Work out the finished part from the listing and answer in its coordinate system (mm). Face numbers are marked on the shaded views. Coordinates: 2 decimals unless noted, no trailing zeros. Loops run counter-clockwise (first coordinate to the right, second up) from the corner with the lowest first, then second, coordinate; pieces in that order, holes last. Notation, with made-up numbers: (-7, 12) - (2, 12) arc R17 ccw to (2, 31) - close; hole circle Ø5 at (-12, 14.5). An arc over 180 degrees is marked (long way). Write each question's results on one line, items separated by ' | '. Start each with the question number.
Item 1: Each of these flat-tipped pins is pushed along its axis until it touches: pin 1 Ø4 at (x, y) = (-15, 9.5) entering from -Z; pin 2 Ø6 at (x, z) = (-18.5, 34) entering from -Y; pin 3 Ø5 at (x, z) = (2, 77) entering from +Y. Where does it stop, or does it pass through?
Item 2: Section A-A, the plane z = 7.5 is taken. Write down the section's boundary in (x, y), plus the area to 3 significant figures.
Item 3: For a pull along X with two mould halves and no side action, classify the marked faces 1, 2 and 3 as +X half, -X half, draft (parallel to the pull), parting line (faces both ways), or undercut.
Item 4: Consider probe 1 along Y at (x, z) = (0, 15); probe 2 along X at (y, z) = (-1, 62); probe 3 along Y at (x, z) = (0, 92). Determine where each line is inside the solid, lowest interval first. Write a range as [from, to].
from build123d import *

# Parameters (mm, degrees)
F3_R = 5.08


# Not quite as in the source:
# - a fillet or chamfer that OpenCascade refuses, or shapes differently, is made with other operations: its cross-section is extruded or revolved along the edge and cut away or added


with BuildPart() as f1:
    # F0 (on Front) → F1 (revolve)
    with BuildSketch(Plane.XZ):
        with BuildLine():
            Line((-26.2792315334, 0), (-22.2152307564, 0))
            Line((-22.2152307564, 0), (-22.2152307564, 66.6416212916))
            ThreePointArc((-22.2152307564, 66.6416212916), (-20.0328257832, 76.8506354666), (-13.8671085173, 85.2750519145))
            Line((-13.8671085173, 85.2750519145), (-13.8671085173, 99.4861274958))
            Line((-13.8671085173, 99.4861274958), (-17.9311092943, 99.4861274958))
            Line((-17.9311092943, 99.4861274958), (-17.9311092943, 87.0146006346))
            ThreePointArc((-17.9311092943, 87.0146006346), (-24.1112579421, 77.6501342728), (-26.2792315334, 66.6416212916))
            Line((-26.2792315334, 66.6416212916), (-26.2792315334, 0))
        make_face()
    revolve(axis=Axis((0, 0, 49.7430637479), (0, 0, -1)))

    # F2: fillet of radius 5.08 on 1 edges, made by hand

    # F2_s1 → F2_t2 (revolve, cut)
    with BuildSketch(Plane.XZ):
        with BuildLine():
            ThreePointArc((-26.2796315334, 4.9781517325), (-25.134523883, 1.7647190024), (-22.2153108172, -0.0003919059))
            Line((-22.2153108172, -0.0003919059), (-22.3170153141, -0.4982462698))
            ThreePointArc((-22.3170153141, -0.4982462698), (-24.2472711753, -0.5081365685), (-26.2792315334, -0.5081365685))
            Line((-26.2792315334, -0.5081365685), (-26.787368102, 0))
            ThreePointArc((-26.787368102, 0), (-26.787368102, 2.4890758662), (-26.787768102, 4.9781517325))
            Line((-26.787768102, 4.9781517325), (-26.2796315334, 4.9781517325))
        make_face()
    revolve(axis=Axis((0, 0, 0), (0, 0, -1)), mode=Mode.SUBTRACT)

    # F3
    f3_edges = [f1.edges().sort_by_distance(p)[0] for p in [
        (17.931109, 0, 87.014601),
    ]]
    fillet(f3_edges, radius=F3_R)


solid = f1.part
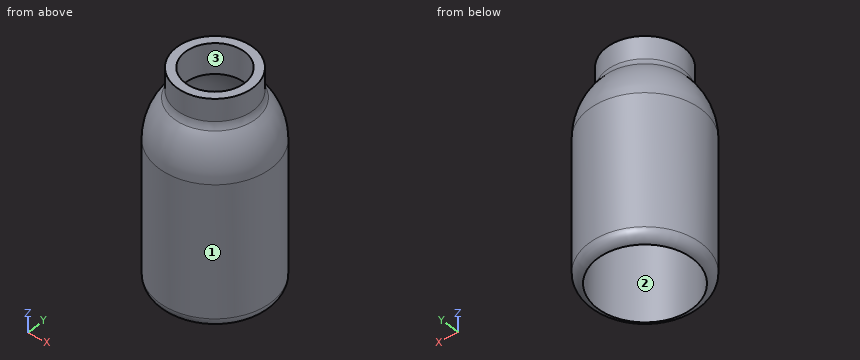
Answer key:
1) pin 1: stops at z = 77.45 | pin 2: stops at y = -21.22 | pin 3: stops at y = 25.14
2) outline: circle Ø52.56 at (0, 0); hole circle Ø44.43 at (0, 0) | area: 619 mm^2
3) face 1: parting line | face 2: undercut | face 3: undercut
4) probe 1: y = [-26.28, -22.22], [22.22, 26.28] | probe 2: x = [-26.26, -22.19], [22.19, 26.26] | probe 3: y = [-17.93, -13.87], [13.87, 17.93]
